from build123d import *

# Parameters (mm, degrees)
PROFILE_R   = 6
PROFILE_R_2 = 3.95


with BuildPart() as part:
    # Tube: sweep along a curve in space
    with BuildLine() as tube_path:
        Line((-140, 103.05702305, 59.5), (-115.387400297, 103.05702305, 59.5))
        Line((-115.387400297, 103.05702305, 59.5), (-110.735387898, 103.067925477, 59.394421789))
        Line((-110.735387898, 103.067925477, 59.394421789), (-106.093057124, 103.100610068, 59.077906882))
        Line((-106.093057124, 103.100610068, 59.077906882), (-101.470069452, 103.155008801, 58.551114001))
        Line((-101.470069452, 103.155008801, 58.551114001), (-96.876046101, 103.231008462, 57.81513949))
        Line((-96.876046101, 103.231008462, 57.81513949), (-92.320548011, 103.328450885, 56.871515038))
        Line((-92.320548011, 103.328450885, 56.871515038), (-87.813055945, 103.447133273, 55.722204485))
        Line((-87.813055945, 103.447133273, 55.722204485), (-83.362950757, 103.586808631, 54.369599743))
        Line((-83.362950757, 103.586808631, 54.369599743), (-78.979493869, 103.747186268, 52.81651581))
        Line((-78.979493869, 103.747186268, 52.81651581), (-74.671807996, 103.927932413, 51.066184917))
        Line((-74.671807996, 103.927932413, 51.066184917), (-70.448858163, 104.128670902, 49.122249798))
        Line((-70.448858163, 104.128670902, 49.122249798), (-69.551141837, 104.173925677, 48.684006254))
        Line((-69.551141837, 104.173925677, 48.684006254), (-65.328192004, 104.374664166, 46.740071136))
        Line((-65.328192004, 104.374664166, 46.740071136), (-61.020506131, 104.55541031, 44.989740243))
        Line((-61.020506131, 104.55541031, 44.989740243), (-56.637049243, 104.715787948, 43.43665631))
        Line((-56.637049243, 104.715787948, 43.43665631), (-52.186944055, 104.855463305, 42.084051567))
        Line((-52.186944055, 104.855463305, 42.084051567), (-47.679451989, 104.974145694, 40.934741015))
        Line((-47.679451989, 104.974145694, 40.934741015), (-43.123953899, 105.071588116, 39.991116562))
        Line((-43.123953899, 105.071588116, 39.991116562), (-38.529930548, 105.147587778, 39.255142051))
        Line((-38.529930548, 105.147587778, 39.255142051), (-33.906942876, 105.20198651, 38.72834917))
        Line((-33.906942876, 105.20198651, 38.72834917), (-29.264612102, 105.234671101, 38.411834263))
        Line((-29.264612102, 105.234671101, 38.411834263), (-24.612599703, 105.245573528, 38.306256052))
        Line((-24.612599703, 105.245573528, 38.306256052), (0, 105.245573528, 38.306256052))
    # Profile → Tube (sweep)
    with BuildSketch(Plane(origin=(-140, 0, 0), x_dir=(0, 0, -1), z_dir=(1, 0, 0))):
        with Locations((-59.5, 103.05702305)):
            Circle(PROFILE_R)
        with Locations((-59.5, 103.05702305)):
            Circle(PROFILE_R_2, mode=Mode.SUBTRACT)
    sweep(path=tube_path.line, transition=Transition.RIGHT)


solid = part.part
Here's how the part is built. I have some questions about the finished solid (model axes, mm). A direction names the side the tool comes from. Coordinates: 2 decimals unless noted, no trailing zeros. Write each loop counter-clockwise with the first axis right and the second up, starting at its lowest first coordinate (ties: lowest second). Pieces come first, ordered by that corner, then holes.
1) Thinking about a two-plate mould opening in Z: for faces 3 (the face through (-59.62, 107.953, 42.22)), 4 (the face through (-140, 104.31, 63.42)), 5 (the face through (-51.36, 106.7, 35.96)), which applies, +Z half, -Z half, draft (parallel to the pull), parting line (faces both ways), or undercut?
Filled in:
face 3: undercut
face 4: draft
face 5: parting line
2) If we section it at A-A (x = -127): List the corners of the cut face in (y, z) for me, plus the area to 3 significant figures.
Filled in:
outline: circle Ø12 at (103.06, 59.5); hole circle Ø7.9 at (103.06, 59.5)
area: 64.1 mm2
3) If I drill on line 1 (Y direction, x = -93, z = 57); line 2 (Y direction, x = -123, z = 59.5); line 3 (Z direction, x = -55.5, y = 105.25), over which ranges is the centre line in solid material (lowest first)?
Filled in:
line 1: y = 97.31 to 99.36, 107.26 to 109.32
line 2: y = 97.06 to 99.11, 107.01 to 109.06
line 3: z = 36.84 to 38.99, 47.19 to 49.37
4) Which directions (+Z, -Z, +X, -X, +Y, -Y) give clear straight access to the entire face, cutting with the end or side of a thin tool? Please do faces 1 (the face through (-56.097, 106.563, 37.283)), 2 (the face through (-12.168, 107.048, 32.583)).
Filled in:
face 1: none
face 2: +X
5) I'm going to push flat-ended pins straight in: pin 1 (5 mm diameter, centred on x = -37, y = 109, fed in from +Z); pin 2 (2 mm diameter, centred on x = -23, y = 103, fed in from +Z); pin 3 (2 mm diameter, centred on x = -73.5, z = 54, fed in from -Y). Where does each tip first touch, or does it pass through?
Filled in:
pin 1: stops at z = 45.04
pin 2: stops at z = 44.18
pin 3: stops at y = 98.32
